```python
from build123d import *

# Parameters (mm, degrees)
SKETCH2_W                = 10
SKETCH2_H                = 86
BOSS_EXTRUDE1_DEPTH      = 10
SKETCH3_W                = 10
SKETCH3_H                = 86
BOSS_EXTRUDE2_DEPTH      = 23
BOSS_EXTRUDE3_REACH      = 246.16
BOSS_EXTRUDE4_DEPTH      = 100
BOSS_EXTRUDE4_DEPTH_BACK = 5
SKETCH5_R                = 47.55
SKETCH7_W                = 10
SKETCH7_H                = 18.447060317
BOSS_EXTRUDE6_DEPTH      = 30
CUT_EXTRUDE2_DEPTH       = 10
BOSS_EXTRUDE7_REACH      = 275.742
SKETCH6_R                = 45.55
CUT_EXTRUDE1_DEPTH       = 100
SKETCH10_W               = 15
SKETCH10_H               = 10
SKETCH10_W_2             = 10
SKETCH10_H_2             = 15
BOSS_EXTRUDE8_DEPTH      = 28.5
FILLET1_R                = 30
FILLET2_R                = 30
FILLET3_R                = 30
SKETCH11_W               = 111.971085125
SKETCH11_H               = 99.425275067
CUT_EXTRUDE3_DEPTH       = 234.52646531


with BuildPart() as part:
    # Sketch2 → Boss-Extrude1 (new body)
    with BuildSketch(Plane(origin=(0, 0, 0), x_dir=(1, 0, 0), z_dir=(0, 1, 0))):
        Polygon((-125, -75), (-115, -75), (-115, -48), (-47, -48), (-47, -75), (47, -75), (47, -48), (115, -48), (115, -75), (125, -75), (125, 75), (115, 75), (115, 48), (47, 48), (47, 75), (-47, 75), (-47, 48), (-115, 48), (-115, 75), (-125, 75), align=None)
        with Locations((-110, 0)):
            Rectangle(SKETCH2_W, SKETCH2_H, mode=Mode.SUBTRACT)
    extrude(amount=BOSS_EXTRUDE1_DEPTH)

    # Sketch3 → Boss-Extrude2 (add)
    with BuildSketch(Plane(origin=(0, 10, 0), x_dir=(1, 0, 0), z_dir=(0, 1, 0))):
        Polygon((-47, 48), (-47, 75), (47, 75), (47, 48), (26, 48), (26, 27), (93, 27), (93, 48), (115, 48), (115, 75), (125, 75), (125, -75), (115, -75), (115, -48), (93, -48), (93, -27), (26, -27), (26, -48), (47, -48), (47, -75), (-47, -75), (-47, -48), (-26, -48), (-26, -27), (-93, -27), (-93, -48), (-115, -48), (-115, -75), (-125, -75), (-125, 75), (-115, 75), (-115, 48), (-93, 48), (-93, 27), (-26, 27), (-26, 48), align=None)
        with Locations((-110, 0)):
            Rectangle(SKETCH3_W, SKETCH3_H, mode=Mode.SUBTRACT)
    extrude(amount=BOSS_EXTRUDE2_DEPTH)

    # Sketch4 → Boss-Extrude3 (add, up to next)
    with BuildSketch(Plane.ZY.offset(105), mode=Mode.PRIVATE) as boss_extrude3_sk1:
        Polygon((-43, 0), (-9.223530158, 14.703891082), (-43, 33), align=None)
    boss_extrude3_tool1 = extrude(boss_extrude3_sk1.sketch, amount=BOSS_EXTRUDE3_REACH, mode=Mode.PRIVATE) - part.part
    # Sketch4 → Boss-Extrude3 (add, up to next)
    with BuildSketch(Plane.ZY.offset(105), mode=Mode.PRIVATE) as boss_extrude3_sk2:
        Polygon((43, 0), (9.223530158, 14.703891082), (-24.552939683, 33), (43, 33), align=None)
    boss_extrude3_tool2 = extrude(boss_extrude3_sk2.sketch, amount=BOSS_EXTRUDE3_REACH, mode=Mode.PRIVATE) - part.part
    add(boss_extrude3_tool1.solids().sort_by_distance((-105, 15.901297, -31.741177))[0])
    add(boss_extrude3_tool2.solids().sort_by_distance((-105, 21.685197, 19.901194))[0])



with BuildPart() as body_2:
    # Sketch5 → Boss-Extrude4 (new, two sides: drawn at the far end of the back side and taken through both)
    with BuildSketch(Plane(origin=(-115, 0, 0), x_dir=(0, 0, -1), z_dir=(1, 0, 0)).offset(-BOSS_EXTRUDE4_DEPTH_BACK)):
        with Locations((0, 80.55)):
            Circle(SKETCH5_R)
    extrude(amount=BOSS_EXTRUDE4_DEPTH + BOSS_EXTRUDE4_DEPTH_BACK)


with BuildPart() as part_1:
    add(part.part)

    add(body_2.part)  # Boss-Extrude6 merges body 2
    # Sketch7 → Boss-Extrude6 (add)
    with BuildSketch(Plane(origin=(0, 33, 0), x_dir=(1, 0, 0), z_dir=(0, 1, 0))):
        Polygon((-120, 0), (-120, 48), (-93, 48), (-93, 27), (-15, 27), (-15, -27), (-93, -27), (-93, -48), (-120, -48), align=None)
        with Locations((-110, 33.776469842)):
            Rectangle(SKETCH7_W, SKETCH7_H, mode=Mode.SUBTRACT)
    extrude(amount=BOSS_EXTRUDE6_DEPTH)

    # Sketch8 → Cut-Extrude2 (cut)
    with BuildSketch(Plane.ZY.offset(105)):
        Polygon((-43, 46.626077643), (-41.871641374, 62.212018017), (-24.552939683, 62.212018017), (-24.552939683, 33), (-43, 33), align=None)
    extrude(amount=CUT_EXTRUDE2_DEPTH, mode=Mode.SUBTRACT)

    # Sketch9 → Boss-Extrude7 (add, up to next)
    with BuildSketch(Plane.ZY.offset(105), mode=Mode.PRIVATE) as boss_extrude7_sk1:
        Polygon((-42.138917347, 58.520153318), (-43, 46.626077643), (-43, 62.212018017), (-41.871641374, 62.212018017), align=None)
    boss_extrude7_tool1 = extrude(boss_extrude7_sk1.sketch, amount=BOSS_EXTRUDE7_REACH, mode=Mode.PRIVATE) - part_1.part
    add(boss_extrude7_tool1.solids().sort_by_distance((-105, 57.016705, -42.62388))[0])

    # Sketch6 → Cut-Extrude1 (cut)
    with BuildSketch(Plane(origin=(-15, 0, 0), x_dir=(0, 0, -1), z_dir=(1, 0, 0))):
        with Locations((0, 80.55)):
            Circle(SKETCH6_R)
    extrude(amount=-CUT_EXTRUDE1_DEPTH, mode=Mode.SUBTRACT)

    # Sketch10 → Boss-Extrude8 (add)
    with BuildSketch(Plane(origin=(0, 33, 0), x_dir=(1, 0, 0), z_dir=(0, 1, 0))):
        with Locations((12.5, 39)):
            Rectangle(SKETCH10_W, SKETCH10_H)
        with Locations((12.5, -39)):
            Rectangle(SKETCH10_W, SKETCH10_H)
        with Locations((63, 0)):
            Rectangle(SKETCH10_W_2, SKETCH10_H_2)
    extrude(amount=BOSS_EXTRUDE8_DEPTH)

    # Fillet1
    # the kernel refuses this fillet: 30 mm, written as the material it adds along each edge
    with BuildSketch(Plane(origin=(5, 33, 44), x_dir=(0, 0, 1), z_dir=(1, 0, 0))) as fillet1_piece_1:
        with BuildLine():
            CenterArc((29.962476533, -30), FILLET1_R, 90, 87.134016017)
            Line((0, -28.5), (0, 0))
            Line((0, 0), (29.962476533, 0))
        make_face()
    extrude(amount=15)

    # Fillet2
    # the kernel refuses this fillet: 30 mm, written as the material it adds along each edge
    with BuildSketch(Plane(origin=(20, 33, -44), x_dir=(0, 0, -1), z_dir=(-1, 0, 0))) as fillet2_piece_1:
        with BuildLine():
            CenterArc((29.962476533, -30), FILLET2_R, 90, 87.134016017)
            Line((0, -28.5), (0, 0))
            Line((0, 0), (29.962476533, 0))
        make_face()
    extrude(amount=15)

    # Fillet3
    # the kernel refuses this fillet: 30 mm, written as the material it adds along each edge
    with BuildSketch(Plane(origin=(68, 33, 7.5), x_dir=(1, 0, 0), z_dir=(0, 0, -1))) as fillet3_piece_1:
        with BuildLine():
            CenterArc((29.962476533, -30), FILLET3_R, 90, 87.134016017)
            Line((0, -28.5), (0, 0))
            Line((0, 0), (29.962476533, 0))
        make_face()
    extrude(amount=15)

    # Sketch11 → Cut-Extrude3 (cut, through all)
    with BuildSketch(Plane.XY.offset(75)):
        with Locations((-64.014457438, 82.712637534)):
            Rectangle(SKETCH11_W, SKETCH11_H)
    extrude(amount=-CUT_EXTRUDE3_DEPTH, mode=Mode.SUBTRACT)


solid = part_1.part
```
CAD build for the part. Positions are in the model's coordinates, mm. A direction names the side the tool comes from. Coordinates: 2 decimals unless noted, no trailing zeros. Order: outer loops, then holes, each group sorted by start corner. A loop starts at its lowest first (then second) coordinate and runs counter-clockwise, first axis right, second up. Notation, with made-up numbers: (-28, -13) - (18, -13) arc R12 ccw to (18, 2) - close; hole circle Ø11 at (45.25, 7.5). An arc over 180 degrees is marked (long way). Answer in a Markdown table with one row per item.
1. Pull direction Z, two halves, no side cores. Call faces 1 (the face through (12, 47, 34)), 2 (the face through (1, 16, 75)), 3 (the face through (47, 16, 61)): +Z half, -Z half, draft (parallel to the pull), parting line (faces both ways), or undercut.
Answer:
| item | result |
|---|---|
| face 1 | undercut |
| face 2 | +Z half |
| face 3 | draft |
2. Flat gauge pins, fed straight in: P1, Ø14, axis at y = 45, z = 50.5, coming from the +X side; P2, Ø6, axis at x = 68, z = 45.5, coming from the +Y side; P3, Ø8, axis at x = 8.5, y = 52.5, coming from the -Z side. Where does each tip first touch, or does it go through?
Answer:
| item | result |
|---|---|
| P1 | x = 20 |
| P2 | y = 10 |
| P3 | z = -47.7 |
3. Slice it at D-D, the plane z = 31.5. List the corners of the cut face in (x, y).
Answer:
| item | result |
|---|---|
| outline | (-125, 0) - (-115, 0) - (-115, 5.01) - (-105, 5.01) - (-105, 0) - (125, 0) - (125, 33) - (93, 33) - (93, 10) - (26, 10) - (26, 33) - (-26, 33) - (-26, 10) - (-93, 10) - (-93, 33) - (-125, 33) - close |
4. Slice it at C-C, the plane x = 13. List the corners of the cut face in (y, z).
Answer:
| item | result |
|---|---|
| outline | (0, -75) - (33, -75) - (33, -73.96) arc R30 cw to (61.5, -44) - (61.5, -34) - (33, -34) - (33, 34) - (61.5, 34) - (61.5, 44) arc R30 cw to (33, 73.96) - (33, 75) - (0, 75) - close |
5. Slice it at B-B, the plane y = 45. List the corners of the cut face in (x, z), then the cut area to 3 significant figures.
Answer:
| item | result |
|---|---|
| outline | (5, -49.96) - (20, -49.96) - (20, -34) - (5, -34) - close; (5, 34) - (20, 34) - (20, 49.96) - (5, 49.96) - close; (58, -7.5) - (73.96, -7.5) - (73.96, 7.5) - (58, 7.5) - close |
| area | 718 mm² |
6. Drill centre lines: L1, parallel to X at y = 6, z = 65; L2, parallel to X at y = 28.5, z = 34.5; L3, parallel to X at y = 31, z = -33.5. Where is each one in solid material? Low to high. Write a range as from..to.
Answer:
| item | result |
|---|---|
| L1 | -125..-115, -47..47, 115..125 |
| L2 | -125..-93, -26..26, 93..125 |
| L3 | -125..-115, -105..-93, -26..26, 93..125 |
7. Slice it at A-A, the plane z = -65. List the corners of the cut face in (x, y).
Answer:
| item | result |
|---|---|
| outline | (-125, 0) - (-115, 0) - (-115, 33) - (-125, 33) - close; (-47, 0) - (47, 0) - (47, 33) - (20, 33) - (20, 34.37) - (5, 34.37) - (5, 33) - (-47, 33) - close; (115, 0) - (125, 0) - (125, 33) - (115, 33) - close |
8. 3-axis set-ups, long thin cutter, end or side, ignore diameter. For faces 4 (the face through (-109.93, 7.25, -26.35)), 5 (the face through (20, 44, -45)), 6 (the face through (59, 10, 37)): which of +Z, -Z, +X, -X, +Y, -Y reach the whole face in a straight line?
Answer:
| item | result |
|---|---|
| face 4 | -Y |
| face 5 | +Z, -Z, +X, +Y |
| face 6 | +Y |
